Source: CAD feature listing. Evaluate the final solid. Frame: model axes, mm. Face numbers are marked on the shaded views. A direction names the side the tool comes from. Round coordinates to 2 decimals unless told otherwise and drop trailing zeros. Write each loop counter-clockwise with the first axis right and the second up, starting at its lowest first coordinate (ties: lowest second). Pieces come first, ordered by that corner, then holes. Notation, with made-up numbers: (80, 3.5) -> (131, 3.5) arc R25 ccw to (131, 23.5) -> close; hole circle Ø3 at (32, -32). An arc over 180 degrees is marked (long way). Put each result on its own line as item: value.
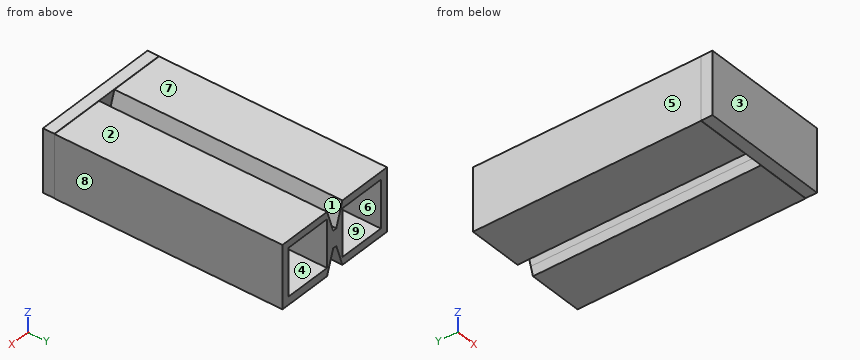
```python
from build123d import *

# Parameters (mm, degrees)
F0_W     = 31.75
F0_H     = 5.3823811583
F0_W_2   = 2.54
F0_H_2   = 11.4322254079
F0_W_3   = 5.08
F0_H_3   = 5.08
F0_H_4   = 31.75
F1_DEPTH = 152.4
F3_W     = 86.36
F3_H     = 41.91
F4_DEPTH = 7.62


with BuildPart() as f1:
    # F0 (on Front) → F1 (new body)
    with BuildSketch(Plane.XZ):
        with Locations((20.955, 5.9824082972)):
            Rectangle(F0_W, F0_H)
        with Locations((-1.27, 24.2451050141)):
            Rectangle(F0_W_2, F0_H_2)
        Polygon((5.08, 45.2012177181), (0, 29.9612177181), (5.08, 29.9612177181), (5.08, 40.4235988763), align=None)
        Polygon((41.91, 45.2012177181), (5.08, 45.2012177181), (5.08, 40.4235988763), (36.83, 40.4235988763), (36.83, 8.6735988763), (41.91, 8.6735988763), align=None)
        with Locations((39.37, 5.9824082972)):
            Rectangle(F0_W_3, F0_H)
        with Locations((-5.08, 24.2451050141)):
            Rectangle(F0_W_3, F0_H_2)
        with Locations((-23.495, 42.6612177181)):
            Rectangle(F0_W, F0_H_3)
        with Locations((-41.91, 42.6612177181)):
            Rectangle(F0_W_3, F0_H_3)
        with Locations((-41.91, 24.2462177181)):
            Rectangle(F0_W_3, F0_H_4)
        with Locations((-41.91, 5.8312177181)):
            Rectangle(F0_W_3, F0_H_3)
        with Locations((-23.495, 5.8312177181)):
            Rectangle(F0_W, F0_H_3)
        Polygon((-7.62, 18.5289923102), (-7.62, 8.3712177181), (-7.62, 3.2912177181), (-2.54, 18.5289923102), align=None)
        with Locations((2.54, 24.2451050141)):
            Rectangle(F0_W_3, F0_H_2)
        Polygon((5.08, 8.6735988763), (3.2856109231, 8.6735988763), (5.08, 3.2912177181), align=None)
        Polygon((5.08, 18.5289923102), (0, 18.5289923102), (3.2856109231, 8.6735988763), (5.08, 8.6735988763), align=None)
        Polygon((-7.62, 45.2012177181), (-7.62, 40.1212177181), (-7.62, 29.9612177181), (-2.54, 29.9612177181), align=None)
    extrude(amount=F1_DEPTH)

    # F3 (on offset) → F4 (join)
    with BuildSketch(Plane.XZ.offset(152.4)):
        with Locations((-1.2090988457, 24.44053792)):
            Rectangle(F3_W, F3_H)
    extrude(amount=F4_DEPTH)


solid = f1.part
```
Q1. Pin query (flat end, axial travel): pin 1 (2.5 mm diameter, centred on x = -14.5, y = -156.5, fed in from -Z); pin 2 (21 mm diameter, centred on x = -21, z = 29, fed in from +Y); pin 3 (12 mm diameter, centred on y = -54.5, z = 25.5, fed in from +X). Return the tip coordinate at first contact, or that it passes through.
Ans:
pin 1: stops at z = 3.49
pin 2: stops at y = -152.4
pin 3: stops at x = 41.91
Q2. Cut plane C-C on z = 25. Output: boundary loops of the cut face in (x, y).
Ans:
outline: (-44.45, -152.4) -> (-44.39, -152.4) -> (-44.39, -160.02) -> (41.97, -160.02) -> (41.97, -152.4) -> (41.91, -152.4) -> (41.91, 0) -> (36.83, 0) -> (36.83, -152.4) -> (5.08, -152.4) -> (5.08, 0) -> (-7.62, 0) -> (-7.62, -152.4) -> (-39.37, -152.4) -> (-39.37, 0) -> (-44.45, 0) -> close
Q3. Cut plane B-B on x = 23. Output: boundary loops of the cut face in (y, z).
Ans:
outline: (-160.02, 3.49) -> (-152.4, 3.49) -> (-152.4, 3.29) -> (0, 3.29) -> (0, 8.67) -> (-152.4, 8.67) -> (-152.4, 40.42) -> (0, 40.42) -> (0, 45.2) -> (-152.4, 45.2) -> (-152.4, 45.4) -> (-160.02, 45.4) -> close
Q4. Reachability of the marked faces 1, 2, 3, 4 and 5 from +Z, -Z, +X, -X, +Y, -Y: full face, straight path, thin tool, end or side. Return the list, or none.
Ans:
face 1: +Z, +Y
face 2: +Z, +X, -X, +Y
face 3: +Z, -Z, +X, -X, -Y
face 4: +Y
face 5: +Z, -Z, -X, +Y, -Y
Q5. Cut plane A-A on y = -60.5. Output: boundary loops of the cut face in (x, z), and give its area (3 significant figures).
Ans:
outline: (-44.45, 3.29) -> (-7.62, 3.29) -> (-2.54, 18.53) -> (0, 18.53) -> (5.08, 3.29) -> (41.91, 3.29) -> (41.91, 45.2) -> (5.08, 45.2) -> (0, 29.96) -> (-2.54, 29.96) -> (-7.62, 45.2) -> (-44.45, 45.2) -> close; hole (-39.37, 8.37) -> (-7.62, 8.37) -> (-7.62, 40.12) -> (-39.37, 40.12) -> close; hole (5.08, 8.67) -> (36.83, 8.67) -> (36.83, 40.42) -> (5.08, 40.42) -> close
area: 1,370 mm^2
Q6. Draft query along X for the marked faces 6, 7, 8 and 9. Return one class per face: +X half, -X half, draft (parallel to the pull), parting line (faces both ways), or undercut.
Ans:
face 6: undercut
face 7: draft
face 8: +X half
face 9: undercut
Q7. Material intervals for line 1 (X direction, y = -79, z = 23.5); line 2 (Z direction, x = 9, y = -62); line 3 (Z direction, x = -31, y = -18), sorted ascending. Write a range as [from, to].
Ans:
line 1: x = [-44.45, -39.37], [-7.62, 5.08], [36.83, 41.91]
line 2: z = [3.29, 8.67], [40.42, 45.2]
line 3: z = [3.29, 8.37], [40.12, 45.2]
Q8. Cut plane D-D on z = 11.5. Output: boundary loops of the cut face in (x, y).
Ans:
outline: (-44.45, -152.4) -> (-44.39, -152.4) -> (-44.39, -160.02) -> (41.97, -160.02) -> (41.97, -152.4) -> (41.91, -152.4) -> (41.91, 0) -> (36.83, 0) -> (36.83, -152.4) -> (5.08, -152.4) -> (5.08, 0) -> (2.34, 0) -> (2.34, -152.4) -> (-4.88, -152.4) -> (-4.88, 0) -> (-7.62, 0) -> (-7.62, -152.4) -> (-39.37, -152.4) -> (-39.37, 0) -> (-44.45, 0) -> close
